Here's the drawing with two shaded views (mm, measured from the low corner). I have some questions. Give positions to 0.01 mm unless a question says otherwise; leave off trailing zeros. Use one line per item in the form item = value. Start each with the question number.
1) Suppose I cut it at A-A, the plane z = 11.5. State how many separate pieces and enclosed holes the cut face has, and give its area (3 significant figures).
2) For pin 1 (7 mm diameter, centred on x = 15.875, z = 9.525, fed in from -Y), with a flat end and sliding along its axis, tell me the tip position at first contact or that it passes through.
3) We'd pull the mould along X, two halves only. Please class the marked faces 1, 2 and 3: released by +X, released by -X, zero draft, split by the parting line, or undercut.
4) Please list where these lines run through material, in increasing order: probe 1 along X at (y, z) = (4.5, 16.75); probe 2 along X at (y, z) = (4.5, 8.25); probe 3 along Y at (x, z) = (3.5, 17.25) (1 decimal).
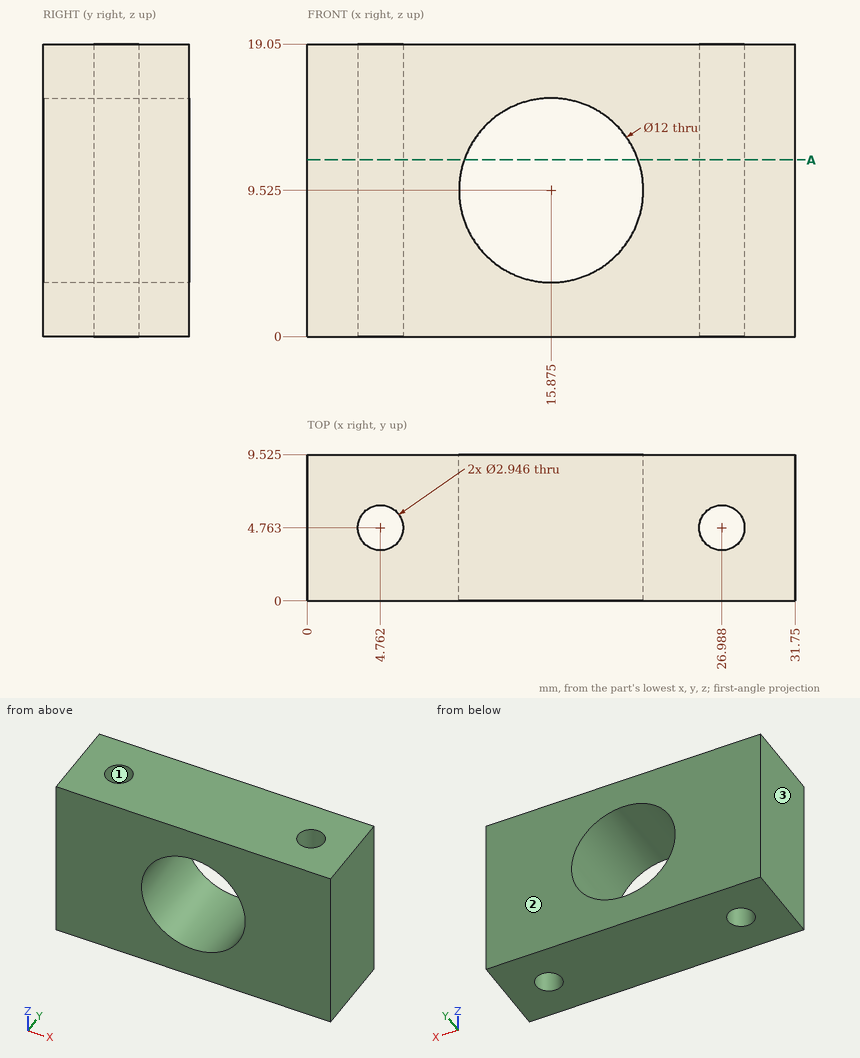
Result sheet:
q1.separate_pieces = 2
q1.enclosed_holes = 2
q1.area = 181 mm²
q2.pin_1 = through
q3.face_1 = undercut
q3.face_2 = zero draft
q3.face_3 = released by -X
q4.probe_1 = 0 to 3.31, 6.21 to 25.54, 28.44 to 31.75
q4.probe_2 = 0 to 3.31, 6.21 to 10.01, 21.74 to 25.54, 28.44 to 31.75
q4.probe_3 = 0 to 4, 5.5 to 9.5
